Work out the finished part from the listing and answer in its coordinate system (mm). Face numbers are marked on the shaded views. A direction names the side the tool comes from. Give positions to 0.01 mm unless a question says otherwise; leave off trailing zeros. Order: outer loops, then holes, each group sorted by start corner. A loop starts at its lowest first (then second) coordinate and runs counter-clockwise, first axis right, second up. Notation, with made-up numbers: (29.25, 49) -> (74.25, 49) arc R28 ccw to (74.25, 78) -> close; hole circle Ø8 at (18, 71). An arc over 180 degrees is marked (long way). Use a Markdown table: item, result. Add a question column.
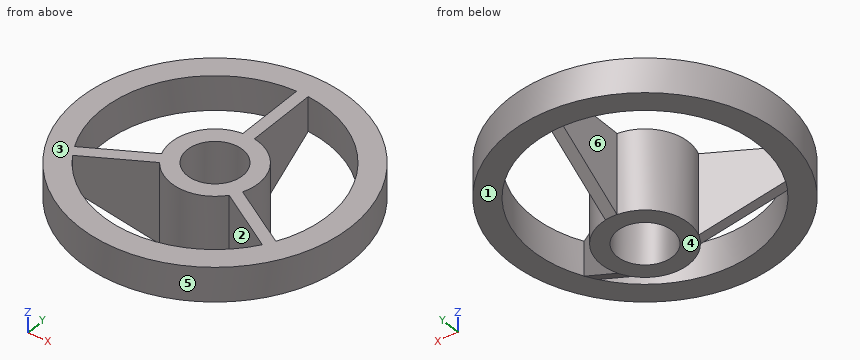
```python
from build123d import *

# Parameters (mm, degrees)
SKETCH1_R           = 1.9
SKETCH1_R_2         = 1.2
BOSS_EXTRUDE1_DEPTH = 3.5
SKETCH2_R           = 5.9
SKETCH2_R_2         = 4.9
BOSS_EXTRUDE2_DEPTH = 1.5
BOSS_EXTRUDE3_DEPTH = 0.25
CIRPATTERN1_COUNT   = 3


with BuildPart() as part:
    # Sketch1 → Boss-Extrude1 (new body)
    with BuildSketch(Plane.XY):
        Circle(SKETCH1_R)
        Circle(SKETCH1_R_2, mode=Mode.SUBTRACT)
    extrude(amount=BOSS_EXTRUDE1_DEPTH)



with BuildPart() as body_2:
    # Sketch2 → Boss-Extrude2 (new body)
    with BuildSketch(Plane.XY.offset(3.5)):
        Circle(SKETCH2_R)
        Circle(SKETCH2_R_2, mode=Mode.SUBTRACT)
    extrude(amount=-BOSS_EXTRUDE2_DEPTH)


with BuildPart() as part_1:
    add(part.part)

    add(body_2.part)  # Boss-Extrude3 merges body 2
    # Sketch3 → Boss-Extrude3 (add, symmetric)
    with BuildSketch(Plane(origin=(0, 0, 0), x_dir=(0, 0, -1), z_dir=(1, 0, 0))):
        Polygon((0, 1.9), (-2, 4.9), (-3.5, 4.9), (-3.5, 1.9), (-3.5, 1.7), (0, 1.7), align=None)
    boss_extrude3 = extrude(amount=BOSS_EXTRUDE3_DEPTH, both=True)

    # CirPattern1: Boss-Extrude3 ×3 about axis
    cirpattern1_axis = Axis((0, 0, 0), (0, 0, 1))
    for i in range(1, CIRPATTERN1_COUNT):
        add(boss_extrude3.rotate(cirpattern1_axis, i * 360 / CIRPATTERN1_COUNT))


solid = part_1.part
```
1) The part is cut by section D-D, the plane z = 2.65. Determine the outline of the cut face in (x, y).
2) Determine the mould class of the marked faces 4, 5 and 6 for opening direction Y: released by +Y, released by -Y, zero draft, split by the parting line, or undercut.
3) The part is cut by section A-A, the plane y = 0. Determine the outline of the cut face in (x, z).
4) The part is cut by section B-B, the plane x = 0. Determine the outline of the cut face in (y, z), then the cut area to 3 significant figures.
5) Flat-ended cylindrical pins translate along their axes: pin 1 (1.5 mm diameter, centred on y = 3, z = 1.5, fed in from +X); pin 2 (1.5 mm diameter, centred on y = 3.5, z = 0.5, fed in from +X). Find the tip coordinate at first contact, or state that the pin passes through.
6) The part is cut by section C-C, the plane y = -4.5. Determine the outline of the cut face in (x, z).
7) Which of the six approach directions +Z, -Z, +X, -X, +Y, -Y give full straight-line access (tool end or side, diameter ignored) to the marked faces 1, 2 and 3?
8) Straight lines are drawn through the part: line 1 (X direction, y = 4.5, z = 2.15); line 2 (X direction, y = 4.25, z = 2.4); line 3 (Y direction, x = -2.5, z = 2.45). For each, find the intervals that lie inside material, in ascending order.
A:
| question | item | result |
|---|---|---|
| 1 | outline | circle Ø11.8 at (0, 0); hole (-4.36, -2.23) -> (-1.76, -0.73) arc R1.9 cw to (-0.25, 1.88) -> (-0.25, 4.89) arc R4.9 ccw to start; hole (-4.11, -2.66) arc R4.9 ccw to (4.11, -2.66) -> (1.51, -1.16) arc R1.9 cw to (-1.51, -1.16) -> close; hole circle Ø2.4 at (0, 0); hole (0.25, 1.88) arc R1.9 cw to (1.76, -0.73) -> (4.36, -2.23) arc R4.9 ccw to (0.25, 4.89) -> close |
| 2 | face 4 | zero draft |
| 2 | face 5 | split by the parting line |
| 2 | face 6 | undercut |
| 3 | outline | (-5.9, 2) -> (-4.9, 2) -> (-4.9, 3.5) -> (-5.9, 3.5) -> close; (-1.9, 0) -> (-1.2, 0) -> (-1.2, 3.5) -> (-1.9, 3.5) -> close; (1.2, 0) -> (1.9, 0) -> (1.9, 3.5) -> (1.2, 3.5) -> close; (4.9, 2) -> (5.9, 2) -> (5.9, 3.5) -> (4.9, 3.5) -> close |
| 4 | outline | (-5.9, 2) -> (-4.9, 2) -> (-4.9, 3.5) -> (-5.9, 3.5) -> close; (-1.9, 0) -> (-1.2, 0) -> (-1.2, 3.5) -> (-1.9, 3.5) -> close; (1.2, 0) -> (1.9, 0) -> (4.9, 2) -> (5.9, 2) -> (5.9, 3.5) -> (1.2, 3.5) -> close |
| 4 | area | 15.4 mm^2 |
| 5 | pin 1 | x = 5.37 |
| 5 | pin 2 | x = 0.25 |
| 6 | outline | (-3.82, 2) -> (-1.94, 2) -> (-1.94, 3.5) -> (-3.82, 3.5) -> close; (1.94, 2) -> (3.82, 2) -> (3.82, 3.5) -> (1.94, 3.5) -> close |
| 7 | face 1 | -Z |
| 7 | face 2 | +Z, -Z |
| 7 | face 3 | +Z, +X, -X, +Y, -Y |
| 8 | line 1 | -3.82 to -1.94, -0.25 to 0.25, 1.94 to 3.82 |
| 8 | line 2 | -4.09 to -2.44, -0.25 to 0.25, 2.44 to 4.09 |
| 8 | line 3 | -5.34 to -4.21, -1.73 to -1.15, 4.21 to 5.34 |
